Geometry check sheet. Reference: the model listing, model coordinates, mm. A direction names the side the tool comes from. Round coordinates to 2 decimals unless told otherwise and drop trailing zeros. Order: outer loops, then holes, each group sorted by start corner. A loop starts at its lowest first (then second) coordinate and runs counter-clockwise, first axis right, second up. Notation, with made-up numbers: (-6, 73) -> (26, 73) arc R36 ccw to (26, 108) -> close; hole circle Ø8 at (-10, 32.5). An arc over 180 degrees is marked (long way). Use a Markdown table: item, result. Add a question column.
Item 1: Sectioned sample at C-C, the plane z = 33.5. Record the cut outline in (x, y), and give its area (3 significant figures).
Item 2: Set-up check for faces 1 (the cylindrical face through (82.01, 5.24, 21.19)), 2 (the cylindrical face through (3.944, 9.235, 14.596)), 3 (the flat face through (-2, 0, 20)), 4 (the flat face through (41, 53, 20)), 5 (the flat face through (8, 11, 20)): record each of +Z, -Z, +X, -X, +Y, -Y from which the full face is reachable in a straight line by a thin tool's end or side.
Item 3: Gauge pin test, flat ends, axial feed: pin 1 Ø20 at (x, z) = (58, 29) entering from -Y; pin 2 Ø10 at (x, y) = (9, 12) entering from +Z (3 decimals). Record the tip position at first contact, or that the pin passes through.
Item 4: Sectioned sample at B-B, the plane z = 20.2. Record the cut outline in (x, y) (3 decimals).
Item 5: Sectioned sample at A-A, the plane y = 11. Record the cut outline in (x, z) (3 decimals).
Item 6: Mould release check, pull along Y, two halves, no side actions. Record for faces 6 (the flat face through (-3, 27, 20)), 7 (the cylindrical face through (80.49, 7.94, 27.59)), 8 (the flat face through (81, 0, 20)): pulls with the +Y half, pulls with the -Y half, needs draft (parallel to the pull), parting line crosses it, or undercut.
Item 7: Sectioned sample at D-D, the plane x = 57. Record the cut outline in (y, z).
Item 8: Material ranges on probe 1 along Y at (x, z) = (82, 20); probe 2 along Y at (x, z) = (81.8, 25.2); probe 3 along X at (y, z) = (34.5, 26.5), recorded low to high. Write a range as [from, to].
Autodesk Inventor part; units mm, degrees
ref_plane "YZ Plane" through (0, 0, 0) normal (1, 0, 0) x (0, 1, 0)
ref_plane "XZ Plane" through (0, 0, 0) normal (0, 1, 0) x (-1, 0, 0)
ref_plane "XY Plane" through (0, 0, 0) normal (0, 0, 1) x (1, 0, 0)
sketch "Sketch1" plane through (0, 0, 0) normal (0, 0, 1) x (1, 0, 0)
  line L0 (0, 0) -> (0, 50)
  line L1 (0, 50) -> (80, 50)
  line L2 (80, 50) -> (80, 0)
  line L3 (80, 0) -> (83, 0)
  line L4 (83, 0) -> (83, 53)
  line L5 (83, 53) -> (-3, 53)
  line L6 (-3, 53) -> (-3, 0)
  line L7 (-3, 0) -> (0, 0)
  dimension "d0" = 50
  dimension "d1" = 80
  dimension "d2" = 3
  dimension "d3" = 53
  dimension "d4" = 86
extrude "Extrusion1" add sketch "Sketch1" along normal blind 40.4
sketch "Sketch2" plane through (83, 0, 0) normal (1, 0, 0) x (0, 0, -1)
  line L0 (0, 0) -> (-40.4, 0)
  circle A0 centre (-20.2, 16) radius 1.25
  circle A1 centre (-25.2, 11) radius 1.25
  circle A2 centre (-20.2, 6) radius 1.25
  circle A3 centre (-15.2, 11) radius 1.25
  point P0 (-20.2, 11)
  dimension "d9" = 2.5
  dimension "d12" = 360
extrude "Extrusion2" cut sketch "Sketch2" against normal up to surface (3 mm away)
sketch "Sketch3" plane through (0, 0, 0) normal (1, 0, 0) x (0, 0, -1)
  line L0 (0, 0) -> (-40.4, 0)
  circle A0 centre (-20.2, 11) radius 5.875
  dimension "d17" = 11.75
extrude "Extrusion3" add sketch "Sketch3" along normal blind 8
sketch "Sketch4" plane through (80, 0, 0) normal (-1, 0, 0) x (0, 0, 1)
  circle A0 centre (20.2, 6) radius 1.25
  circle A1 centre (20.2, 16) radius 1.25
  circle A2 centre (20.2, 11) radius 8
  point P0 (0, 0)
  dimension "d20" = 16
extrude "Extrusion4" cut sketch "Sketch4" against normal blind 1
properties part number "Tilt_Bracket"
Found:
| question | item | result |
|---|---|---|
| 1 | outline | (-3, 0) -> (0, 0) -> (0, 50) -> (80, 50) -> (80, 0) -> (83, 0) -> (83, 53) -> (-3, 53) -> close |
| 1 | area | 558 mm2 |
| 2 | face 1 | +X |
| 2 | face 2 | none |
| 2 | face 3 | +Z, -Z, +X, -X, -Y |
| 2 | face 4 | +Z, -Z, +X, -X, +Y |
| 2 | face 5 | +Z, -Z, -Y |
| 3 | pin 1 | stops at y = 50 |
| 3 | pin 2 | stops at z = 26.075 |
| 4 | outline | (-3, 0) -> (0, 0) -> (0, 5.125) -> (8, 5.125) -> (8, 16.875) -> (0, 16.875) -> (0, 50) -> (80, 50) -> (80, 19) -> (81, 19) -> (81, 17.25) -> (83, 17.25) -> (83, 53) -> (-3, 53) -> close; (80, 0) -> (83, 0) -> (83, 4.75) -> (81, 4.75) -> (81, 3) -> (80, 3) -> close; (81, 7.25) -> (83, 7.25) -> (83, 14.75) -> (81, 14.75) -> close |
| 5 | outline | (-3, 0) -> (0, 0) -> (0, 14.325) -> (8, 14.325) -> (8, 26.075) -> (0, 26.075) -> (0, 40.4) -> (-3, 40.4) -> close; (80, 0) -> (83, 0) -> (83, 13.95) -> (81, 13.95) -> (81, 12.2) -> (80, 12.2) -> close; (80, 28.2) -> (81, 28.2) -> (81, 26.45) -> (83, 26.45) -> (83, 40.4) -> (80, 40.4) -> close; (81, 16.45) -> (83, 16.45) -> (83, 23.95) -> (81, 23.95) -> close |
| 6 | face 6 | needs draft |
| 6 | face 7 | undercut |
| 6 | face 8 | pulls with the -Y half |
| 7 | outline | (50, 0) -> (53, 0) -> (53, 40.4) -> (50, 40.4) -> close |
| 8 | probe 1 | y = [0, 4.77], [7.23, 14.77], [17.23, 53] |
| 8 | probe 2 | y = [0, 9.75], [12.25, 53] |
| 8 | probe 3 | x = [-3, 0], [80, 83] |
